Work out the finished part from the listing and answer in its coordinate system (mm). Face numbers are marked on the shaded views. A direction names the side the tool comes from. Coordinates: 2 decimals unless noted, no trailing zeros. Loops run counter-clockwise (first coordinate to the right, second up) from the corner with the lowest first, then second, coordinate; pieces in that order, holes last. Notation, with made-up numbers: (39, 64.5) -> (48, 64.5) arc R15 cw to (48, 71.5) -> close; hole circle Ø6 at (86, 32.5). An arc over 180 degrees is marked (long way). Answer as CSV lines item,"result".
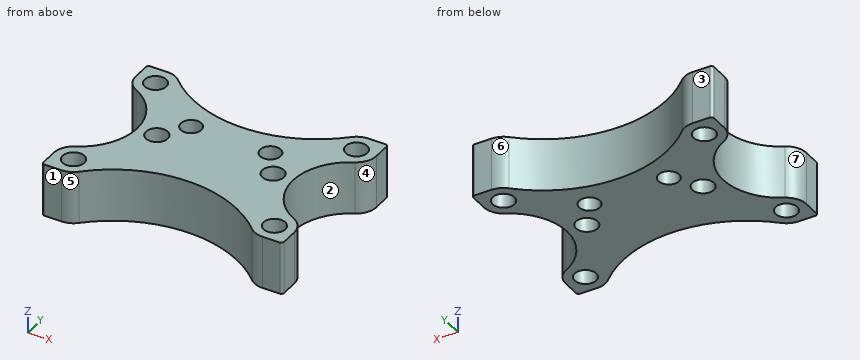
```python
from build123d import *

# Parameters (mm, degrees)
SKETCH1_R           = 2.05
SKETCH1_R_2         = 1.95
BOSS_EXTRUDE1_DEPTH = 10
FILLET1_R           = 0.5


with BuildPart() as part:
    # Sketch1 → Boss-Extrude1 (new body)
    with BuildSketch(Plane.XY):
        with BuildLine():
            Line((-19, 16.75), (-22.75, 16.75))
            Line((-22.75, 16.75), (-22.75, 13))
            ThreePointArc((-22.75, 13), (-22.193718688, 11.034634654), (-20.689914163, 9.652360515))
            ThreePointArc((-20.689914163, 9.652360515), (-14.75, 0), (-20.689914163, -9.652360515))
            ThreePointArc((-20.689914163, -9.652360515), (-22.193718688, -11.034634654), (-22.75, -13))
            Line((-22.75, -13), (-22.75, -16.75))
            Line((-22.75, -16.75), (-19, -16.75))
            ThreePointArc((-19, -16.75), (-17.583685544, -16.472254795), (-16.377170848, -15.680161793))
            ThreePointArc((-16.377170848, -15.680161793), (0, -9), (16.377170848, -15.680161793))
            ThreePointArc((16.377170848, -15.680161793), (17.583685544, -16.472254795), (19, -16.75))
            Line((19, -16.75), (22.75, -16.75))
            Line((22.75, -16.75), (22.75, -13))
            ThreePointArc((22.75, -13), (22.193718688, -11.034634654), (20.689914163, -9.652360515))
            ThreePointArc((20.689914163, -9.652360515), (14.75, 0), (20.689914163, 9.652360515))
            ThreePointArc((20.689914163, 9.652360515), (22.193718688, 11.034634654), (22.75, 13))
            Line((22.75, 13), (22.75, 16.75))
            Line((22.75, 16.75), (19, 16.75))
            ThreePointArc((19, 16.75), (17.583685544, 16.472254795), (16.377170848, 15.680161793))
            ThreePointArc((16.377170848, 15.680161793), (0, 9), (-16.377170848, 15.680161793))
            ThreePointArc((-16.377170848, 15.680161793), (-17.583685544, 16.472254795), (-19, 16.75))
        make_face()
        with Locations((19, 13)):
            Circle(SKETCH1_R, mode=Mode.SUBTRACT)
        with Locations((-19, 13)):
            Circle(SKETCH1_R, mode=Mode.SUBTRACT)
        with Locations((-19, -13)):
            Circle(SKETCH1_R, mode=Mode.SUBTRACT)
        with Locations((19, -13)):
            Circle(SKETCH1_R, mode=Mode.SUBTRACT)
        with Locations((-11, 0)):
            Circle(SKETCH1_R, mode=Mode.SUBTRACT)
        with Locations((11, 0)):
            Circle(SKETCH1_R, mode=Mode.SUBTRACT)
        with Locations(Location((7.5, 5, 0), (0, 0, 180))):
            Circle(SKETCH1_R_2, mode=Mode.SUBTRACT)
        with Locations(Location((-7.5, 5, 0), (0, 0, 180))):
            Circle(SKETCH1_R_2, mode=Mode.SUBTRACT)
    extrude(amount=BOSS_EXTRUDE1_DEPTH)

    # Fillet1
    fillet1_edges = [part.edges().sort_by_distance(p)[0] for p in [
        (22.75, 16.75, 5),
        (22.75, -16.75, 5),
        (-22.75, -16.75, 5),
        (-22.75, 16.75, 5),
    ]]
    fillet(fillet1_edges, radius=FILLET1_R)


solid = part.part
```
(1) Flat-ended cylindrical pins translate along their axes: pin 1 Ø2 at (x, z) = (11, 3) entering from -Y; pin 2 Ø3 at (x, z) = (3.5, 8.5) entering from +Y; pin 3 Ø6 at (y, z) = (-6, 4) entering from -X. Find the tip coordinate at first contact, or state that the pin passes through.
Computed values:
pin 1,"y = -12.31"
pin 2,"y = 9.54"
pin 3,"x = -19.57"
(2) A cutting plane is placed at A-A, the plane y = 0. Write down the section's boundary in (x, z), and give its area (3 significant figures).
Computed values:
outline,"(-14.75, 0) -> (-13.05, 0) -> (-13.05, 10) -> (-14.75, 10) -> close; (-8.95, 0) -> (8.95, 0) -> (8.95, 10) -> (-8.95, 10) -> close; (13.05, 0) -> (14.75, 0) -> (14.75, 10) -> (13.05, 10) -> close"
area,"213 mm2"
(3) A cutting plane is placed at B-B, the plane z = 9. Count the separate pieces of the cut face and the enclosed holes in it, and give its area (3 significant figures).
Computed values:
separate pieces,"1"
enclosed holes,"8"
area,"795 mm2"
(4) A cutting plane is placed at D-D, the plane x = -18. Write down the section's boundary in (y, z).
Computed values:
outline,"(-16.61, 0) -> (-14.79, 0) -> (-14.79, 10) -> (-16.61, 10) -> close; (-11.21, 0) -> (-7.73, 0) -> (-7.73, 10) -> (-11.21, 10) -> close; (7.73, 0) -> (11.21, 0) -> (11.21, 10) -> (7.73, 10) -> close; (14.79, 0) -> (16.61, 0) -> (16.61, 10) -> (14.79, 10) -> close"
(5) A cutting plane is placed at C-C, the plane x = -8. Write down the section's boundary in (y, z), and give its area (3 significant figures).
Computed values:
outline,"(-10.41, 0) -> (3.12, 0) -> (3.12, 10) -> (-10.41, 10) -> close; (6.88, 0) -> (10.41, 0) -> (10.41, 10) -> (6.88, 10) -> close"
area,"170 mm2"
(6) Which of the six approach directions +Z, -Z, +X, -X, +Y, -Y give full straight-line access (tool end or side, diameter ignored) to the marked faces 4, 5, 6 and 7?
Computed values:
face 4,"+Z, -Z, +X"
face 5,"+Z, -Z, -Y"
face 6,"+Z, -Z, +Y"
face 7,"+Z, -Z, -X"
(7) For a pull along Y with two mould halves and no side action, classify the marked faces 1, 2 and 3 as pulls with the +Y half, pulls with the -Y half, needs draft (parallel to the pull), parting line crosses it, or undercut.
Computed values:
face 1,"pulls with the -Y half"
face 2,"undercut"
face 3,"pulls with the +Y half"
(8) Consider line 1 along Y through (x, z) = (19, 2.5); line 2 along X through (y, z) = (14.5, 2); line 3 along X through (y, z) = (5, 6.5). Determine where each line is inside the solid, lowest interval first.
Computed values:
line 1,"-16.75 to -15.05, -10.95 to -8.59, 8.59 to 10.95, 15.05 to 16.75"
line 2,"-22.75 to -20.4, -17.6 to -15.08, 15.08 to 17.6, 20.4 to 22.75"
line 3,"-15.98 to -9.45, -5.55 to 5.55, 9.45 to 15.98"
